Source: CAD feature listing. Evaluate the final solid. Frame: model axes, mm. Face numbers are marked on the shaded views. A direction names the side the tool comes from. Coordinates: 2 decimals unless noted, no trailing zeros. Order: outer loops, then holes, each group sorted by start corner. A loop starts at its lowest first (then second) coordinate and runs counter-clockwise, first axis right, second up. Notation, with made-up numbers: (-35.5, 8.5) -> (-6.5, 8.5) arc R6 cw to (-6.5, 13.5) -> close; hole circle Ø2 at (-7, 70.5). An arc over 180 degrees is marked (long way). Put each result on its own line as item: value.
from build123d import *

# Parameters (mm, degrees)
BOSS_EXTRUDE2_DEPTH = 25
SKETCH4_R           = 8
BOSS_EXTRUDE3_DEPTH = 20
SKETCH5_R           = 7.061522099
CUT_EXTRUDE2_DEPTH  = 36


with BuildPart() as part:
    # Sketch3 → Boss-Extrude2 (new body, symmetric)
    with BuildSketch(Plane.XY):
        Polygon((14.5, -30), (17.5, -30), (17.5, 30), (-17.5, 30), (-17.5, -30), (-14.5, -30), (-14.5, 27), (14.5, 27), align=None)
    extrude(amount=BOSS_EXTRUDE2_DEPTH, both=True)

    # Sketch4 → Boss-Extrude3 (add)
    with BuildSketch(Plane(origin=(0, 30, 0), x_dir=(1, 0, 0), z_dir=(0, 1, 0))):
        Circle(SKETCH4_R)
    extrude(amount=BOSS_EXTRUDE3_DEPTH)

    # Sketch5 → Cut-Extrude2 (cut, through all)
    with BuildSketch(Plane.ZY.offset(17.5)):
        with Locations((-1.403257922, -21.231511185)):
            Circle(SKETCH5_R)
    extrude(amount=-CUT_EXTRUDE2_DEPTH, mode=Mode.SUBTRACT)


solid = part.part
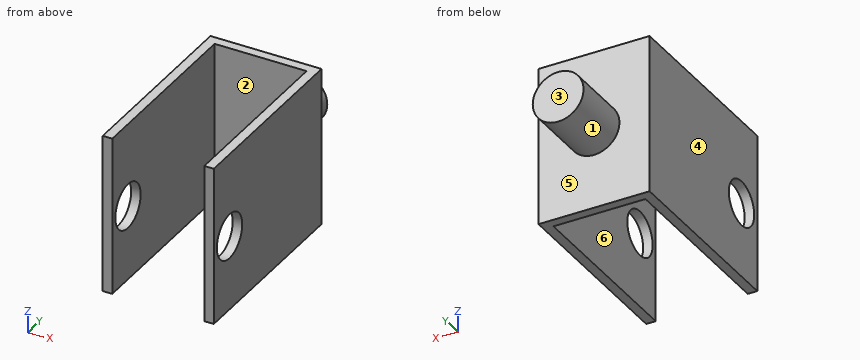
1. Cut plane D-D on z = -1.5. Output: boundary loops of the cut face in (x, y).
Numbers:
outline: (-17.5, -30) -> (-14.5, -30) -> (-14.5, -28.29) -> (-17.5, -28.29) -> close; (-17.5, -14.17) -> (-14.5, -14.17) -> (-14.5, 27) -> (14.5, 27) -> (14.5, -14.17) -> (17.5, -14.17) -> (17.5, 30) -> (7.86, 30) -> (7.86, 50) -> (-7.86, 50) -> (-7.86, 30) -> (-17.5, 30) -> close; (14.5, -30) -> (17.5, -30) -> (17.5, -28.29) -> (14.5, -28.29) -> close
2. Ray query, line 1 along X through (y, z) = (-7.5, -1.5); line 2 along Z through (x, y) = (-15, -21); line 3 along Y through (x, z) = (-3.5, 9.5). Return the intervals inside material, ascending.
Numbers:
line 1: x = -17.5 to -14.5, 14.5 to 17.5
line 2: z = -25 to -8.46, 5.65 to 25
line 3: y = 27 to 30
3. First-contact query: pin 1 (1 mm diameter, centred on x = -13.5, z = 2.5, fed in from -Y); pin 2 (6 mm diameter, centred on x = 9.5, z = -14, fed in from +Y); pin 3 (12.5 mm diameter, centred on y = -21.23, z = -1.4, fed in from +X). Flat tips, straight axial feed; report the tip coordinate or a pass-through.
Numbers:
pin 1: stops at y = 27
pin 2: stops at y = 30
pin 3: passes through
4. Set-up query: the marked faces 1, 2 and 3. Return all of +Z, -Z, +X, -X, +Y, -Y with unobstructed straight access to the full face (end or side cutting, diameter ignored); none if empty.
Numbers:
face 1: +Y
face 2: +Z, -Z, -Y
face 3: +Z, -Z, +X, -X, +Y
5. Cut plane A-A on y = 2. Output: boundary loops of the cut face in (x, z), plus the area to 3 significant figures.
Numbers:
outline: (-17.5, -25) -> (-14.5, -25) -> (-14.5, 25) -> (-17.5, 25) -> close; (14.5, -25) -> (17.5, -25) -> (17.5, 25) -> (14.5, 25) -> close
area: 300 mm2
6. Cut plane B-B on z = -10.5. Output: boundary loops of the cut face in (x, y), plus the area to 3 significant figures.
Numbers:
outline: (-17.5, -30) -> (-14.5, -30) -> (-14.5, 27) -> (14.5, 27) -> (14.5, -30) -> (17.5, -30) -> (17.5, 30) -> (-17.5, 30) -> close
area: 447 mm2
7. Cut plane C-C on x = 0. Output: boundary loops of the cut face in (y, z).
Numbers:
outline: (27, -25) -> (30, -25) -> (30, -8) -> (50, -8) -> (50, 8) -> (30, 8) -> (30, 25) -> (27, 25) -> close
8. Pull-direction query (X, two-part tool) for the marked faces 4, 5 and 6; classes: pulls with the +X half, pulls with the -X half, needs draft (parallel to the pull), parting line crosses it, or undercut.
Numbers:
face 4: pulls with the -X half
face 5: needs draft
face 6: undercut
